```python
from build123d import *

# Parameters (mm, degrees)
SKETCH1_W           = 101.6
SKETCH1_H           = 127
BOSS_EXTRUDE1_DEPTH = 19.05
SKETCH2_W           = 25.4
SKETCH2_H           = 127
CUT_EXTRUDE1_DEPTH  = 6.35
CUT_EXTRUDE2_REACH  = 165.751
SKETCH4_R           = 6.35
SKETCH9_W           = 50.8
SKETCH9_H           = 50.8
CUT_EXTRUDE7_DEPTH  = 6.35
SKETCH11_R          = 3.175
CUT_EXTRUDE8_DEPTH  = 9.525
SKETCH12_R          = 9.525
CUT_EXTRUDE9_DEPTH  = 164.751221369


with BuildPart() as part:
    # Sketch1 → Boss-Extrude1 (new body)
    with BuildSketch(Plane.XY):
        with Locations((50.8, 63.5)):
            Rectangle(SKETCH1_W, SKETCH1_H)
    extrude(amount=BOSS_EXTRUDE1_DEPTH)

    # Sketch2 → Cut-Extrude1 (cut)
    with BuildSketch(Plane(origin=(0, 0, 0), x_dir=(-1, 0, 0), z_dir=(0, 0, -1))):
        with Locations((-88.9, 63.5)):
            Rectangle(SKETCH2_W, SKETCH2_H)
        with Locations((-12.7, 63.5)):
            Rectangle(SKETCH2_W, SKETCH2_H)
    extrude(amount=-CUT_EXTRUDE1_DEPTH, mode=Mode.SUBTRACT)

    # Sketch4 → Cut-Extrude2 (cut, up to next)
    with BuildSketch(Plane.XY.offset(19.05), mode=Mode.PRIVATE) as cut_extrude2_sk1:
        with Locations((12.7, 114.3)):
            Circle(SKETCH4_R)
    cut_extrude2_tool1 = extrude(cut_extrude2_sk1.sketch, amount=-CUT_EXTRUDE2_REACH, mode=Mode.PRIVATE) & part.part
    # Sketch4 → Cut-Extrude2 (cut, up to next)
    with BuildSketch(Plane.XY.offset(19.05), mode=Mode.PRIVATE) as cut_extrude2_sk2:
        with Locations((12.7, 12.7)):
            Circle(SKETCH4_R)
    cut_extrude2_tool2 = extrude(cut_extrude2_sk2.sketch, amount=-CUT_EXTRUDE2_REACH, mode=Mode.PRIVATE) & part.part
    # Sketch4 → Cut-Extrude2 (cut, up to next)
    with BuildSketch(Plane.XY.offset(19.05), mode=Mode.PRIVATE) as cut_extrude2_sk3:
        with Locations(Location((88.9, 12.7, 0), (0, 0, 180))):
            Circle(SKETCH4_R)
    cut_extrude2_tool3 = extrude(cut_extrude2_sk3.sketch, amount=-CUT_EXTRUDE2_REACH, mode=Mode.PRIVATE) & part.part
    # Sketch4 → Cut-Extrude2 (cut, up to next)
    with BuildSketch(Plane.XY.offset(19.05), mode=Mode.PRIVATE) as cut_extrude2_sk4:
        with Locations(Location((88.9, 114.3, 0), (0, 0, 180))):
            Circle(SKETCH4_R)
    cut_extrude2_tool4 = extrude(cut_extrude2_sk4.sketch, amount=-CUT_EXTRUDE2_REACH, mode=Mode.PRIVATE) & part.part
    add(cut_extrude2_tool1.solids().sort_by_distance((12.7, 114.3, 19.05))[0], mode=Mode.SUBTRACT)
    add(cut_extrude2_tool2.solids().sort_by_distance((12.7, 12.7, 19.05))[0], mode=Mode.SUBTRACT)
    add(cut_extrude2_tool3.solids().sort_by_distance((88.9, 12.7, 19.05))[0], mode=Mode.SUBTRACT)
    add(cut_extrude2_tool4.solids().sort_by_distance((88.9, 114.3, 19.05))[0], mode=Mode.SUBTRACT)

    # Sketch9 → Cut-Extrude7 (cut)
    with BuildSketch(Plane(origin=(0, 0, 0), x_dir=(-1, 0, 0), z_dir=(0, 0, -1))):
        with Locations((-50.8, 25.4)):
            Rectangle(SKETCH9_W, SKETCH9_H)
        with Locations((-50.8, 101.6)):
            Rectangle(SKETCH9_W, SKETCH9_H)
    extrude(amount=-CUT_EXTRUDE7_DEPTH, mode=Mode.SUBTRACT)

    # Sketch11 → Cut-Extrude8 (cut)
    with BuildSketch(Plane.XY.offset(19.05)):
        with Locations((50.8, 63.5)):
            Circle(SKETCH11_R)
    extrude(amount=-CUT_EXTRUDE8_DEPTH, mode=Mode.SUBTRACT)

    # Sketch12 → Cut-Extrude9 (cut, through all)
    with BuildSketch(Plane.XY.offset(19.05)):
        with Locations((12.7, 114.3)):
            Circle(SKETCH12_R)
        with Locations((88.9, 114.3)):
            Circle(SKETCH12_R)
        with Locations((12.7, 12.7)):
            Circle(SKETCH12_R)
        with Locations((88.9, 12.7)):
            Circle(SKETCH12_R)
        with Locations((88.632472784, -89.675466105)):
            Circle(SKETCH12_R)
    extrude(amount=-CUT_EXTRUDE9_DEPTH, mode=Mode.SUBTRACT)


solid = part.part
```
Input: part model. Units: mm. Frame: model coordinates. A direction names the side the tool comes from. Round coordinates to 2 decimals unless told otherwise and drop trailing zeros. Write each loop counter-clockwise with the first axis right and the second up, starting at its lowest first coordinate (ties: lowest second). Pieces come first, ordered by that corner, then holes. Notation, with made-up numbers: M -26,35.25 L -13,35.25 A30 ccw -13,66.25 Z; hole C -31,-18.75 d7. An arc over 180 degrees is marked long. Write each question's results on one line, items separated by ' | '.
Q1. Section query D-D (x = 8.5). Return loops of the section in (y, z).
Results:
outline: M 0,6.35 L 4.15,6.35 L 4.15,19.05 L 0,19.05 Z; M 21.25,6.35 L 105.75,6.35 L 105.75,19.05 L 21.25,19.05 Z; M 122.85,6.35 L 127,6.35 L 127,19.05 L 122.85,19.05 Z
Q2. Pin query (flat end, axial travel): P1, Ø1.9, axis at x = 50.5, y = 64.5, coming from the +Z side (3 decimals); P2, Ø3, axis at y = 67, z = 2.5, coming from the +X side; P3, Ø2, axis at y = 103, z = 5, coming from the +X side; P4, Ø3, axis at x = 52, z = 1.5, coming from the -Y side. Return the tip coordinate at first contact, or that it passes through.
Results:
P1: stops at z = 9.525 | P2: stops at x = 76.2 | P3: passes through | P4: stops at y = 50.8
Q3. Section query B-B (z = 8). Return loops of the section in (x, y) (3 decimals).
Results:
outline: M 0,0 L 101.6,0 L 101.6,127 L 0,127 Z; hole C 12.7,12.7 d19.05; hole C 12.7,114.3 d19.05; hole C 88.9,12.7 d19.05; hole C 88.9,114.3 d19.05
Q4. Line query: line 1 along Y through (x, z) = (12.7, 14.75) (3 decimals); line 2 along Y through (x, z) = (50.8, 12.5) (3 decimals); line 3 along X through (y, z) = (18, 16.5). Output: solid intervals per line, ascending.
Results:
line 1: y = 0 to 3.175, 22.225 to 104.775, 123.825 to 127 | line 2: y = 0 to 60.325, 66.675 to 127 | line 3: x = 0 to 4.79, 20.61 to 80.99, 96.81 to 101.6
Q5. Access query for faces 5 (the face through (51, 50.8, 3)), 6 (the face through (53.83, 64.45, 14.35)), 7 (the face through (101.6, 63, 13)), 8 (the face through (25.4, 63, 3)), 9 (the face through (76.2, 63, 3)). Directions: +Z, -Z, +X, -X, +Y, -Y. A direction counts if a zero-diameter tool reaches every point of the face in a straight line with its end or side. Return the directions, or none.
Results:
face 5: -Z, +X, -X, -Y | face 6: +Z | face 7: +Z, -Z, +X, +Y, -Y | face 8: -Z, -X, +Y, -Y | face 9: -Z, +X, +Y, -Y
Q6. Draft query along Y for faces 1 (the face through (51, 76.2, 3)), 2 (the face through (81.88, 120.74, 12.79)), 3 (the face through (10.64, 3.4, 12.79)), 4 (the face through (50, 64, 0)). Return one class per face: released by +Y, released by -Y, zero draft, split by the parting line, or undercut.
Results:
face 1: released by +Y | face 2: undercut | face 3: undercut | face 4: zero draft
Q7. Section query A-A (y = 114.3). Return loops of the section in (x, z) (3 decimals), and give its area (3 significant figures).
Results:
outline: M 0,6.35 L 3.175,6.35 L 3.175,19.05 L 0,19.05 Z; M 22.225,6.35 L 79.375,6.35 L 79.375,19.05 L 22.225,19.05 Z; M 98.425,6.35 L 101.6,6.35 L 101.6,19.05 L 98.425,19.05 Z | area: 806 mm^2
Q8. Section query C-C (x = 62). Return loops of the section in (y, z).
Results:
outline: M 0,6.35 L 50.8,6.35 L 50.8,0 L 76.2,0 L 76.2,6.35 L 127,6.35 L 127,19.05 L 0,19.05 Z
